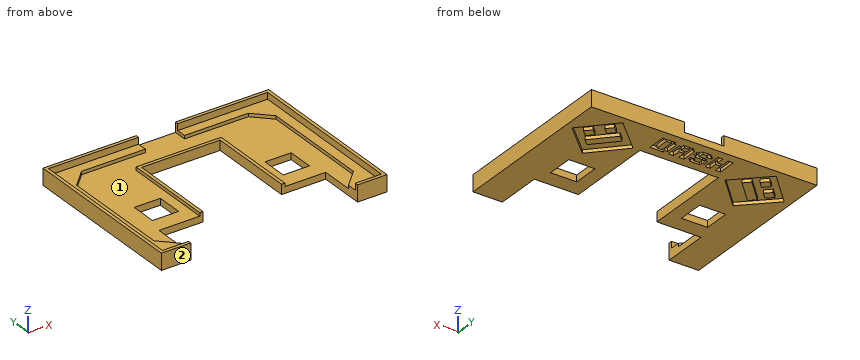
from build123d import *

# Parameters (mm, degrees)
SKICA1_W                    = 67
SKICA1_H                    = 50
P_IDAT_VYSUNUT_M1_DEPTH     = 3
ODEBRAT_VYSUNUT_M1_DEPTH    = 1
SKICA3_W                    = 8
SKICA3_H                    = 8
ODEBRAT_VYSUNUT_M2_DEPTH    = 4
VYSUNOUT_TENKOST_NN_1_DEPTH = 1
VYSUNOUT_TENKOST_NN_2_DEPTH = 5
SKICA6_W                    = 12
SKICA6_H                    = 4
ODEBRAT_VYSUNUT_M3_DEPTH    = 4
ODEBRAT_VYSUNUT_M5_DEPTH    = 1
P_IDAT_START                = -1
P_IDAT_VYSUNUT_M3_DEPTH     = 1
ODEBRAT_VYSUNUT_M7_DEPTH    = 1
SKICA10_W                   = 1.6
SKICA10_H                   = 4
SKICA10_H_2                 = 1.6
P_IDAT_VYSUNUT_M4_DEPTH     = 1


with BuildPart() as part:
    # Skica1 → Přidat vysunutím1 (new body)
    with BuildSketch(Plane.XY):
        Rectangle(SKICA1_W, SKICA1_H)
    extrude(amount=P_IDAT_VYSUNUT_M1_DEPTH)

    # Skica2 → Odebrat vysunutím1 (cut)
    with BuildSketch(Plane.XY.offset(3)):
        Polygon((-25.5, -22), (-30.5, -17), (-30.5, 17), (-25.5, 22), (25.5, 22), (30.5, 17), (30.5, -17), (25.5, -22), align=None)
    extrude(amount=-ODEBRAT_VYSUNUT_M1_DEPTH, mode=Mode.SUBTRACT)

    # Skica3 → Odebrat vysunutím2 (cut, through all)
    with BuildSketch(Plane(origin=(0, 0, 0), x_dir=(-1, 0, 0), z_dir=(0, 0, -1))):
        with Locations((20, -3)):
            Rectangle(SKICA3_W, SKICA3_H)
        with Locations((-20, -3)):
            Rectangle(SKICA3_W, SKICA3_H)
        Polygon((25.5, -25), (-25.5, -25), (-25.5, -12), (-12, -12), (-12, 15), (12, 15), (12, -12), (25.5, -12), align=None)
    extrude(amount=-ODEBRAT_VYSUNUT_M2_DEPTH, mode=Mode.SUBTRACT)

    # Skica4 → Vysunout tenkostěnný1 (add)
    with BuildSketch(Plane.XY.offset(2)):
        Polygon((-12, -12), (-12, 15), (12, 15), (12, -12), (13, -12), (13, 16), (-13, 16), (-13, -12), align=None)
    extrude(amount=VYSUNOUT_TENKOST_NN_1_DEPTH)

    # Skica5 → Vysunout tenkostěnný2 (add)
    with BuildSketch(Plane(origin=(0, 0, 0), x_dir=(-1, 0, 0), z_dir=(0, 0, -1))):
        Polygon((-25.5, -25), (-33.5, -25), (-33.5, 25), (33.5, 25), (33.5, -25), (25.5, -25), (25.5, -26), (34.5, -26), (34.5, 26), (-34.5, 26), (-34.5, -26), (-25.5, -26), align=None)
    extrude(amount=-VYSUNOUT_TENKOST_NN_2_DEPTH)

    # Skica6 → Odebrat vysunutím3 (cut, through all)
    with BuildSketch(Plane.XY.offset(2)):
        with Locations((0, 24)):
            Rectangle(SKICA6_W, SKICA6_H)
    extrude(amount=ODEBRAT_VYSUNUT_M3_DEPTH, mode=Mode.SUBTRACT)

    # Skica7 → Odebrat vysunutím5 (cut)
    with BuildSketch(Plane(origin=(0, 0, 0), x_dir=(-1, 0, 0), z_dir=(0, 0, -1))):
        Polygon((-32.44, 14.540476732), (-23.459523268, 23.94), (-14.06, 14.959523268), (-23.040476732, 5.56), align=None)
        Polygon((14.06, 14.959523268), (23.040476732, 5.56), (32.44, 14.540476732), (23.459523268, 23.94), align=None)
    extrude(amount=-ODEBRAT_VYSUNUT_M5_DEPTH, mode=Mode.SUBTRACT)

    # Skica8 → Přidat vysunutím3 (add)
    with BuildSketch(Plane(origin=(0, 0, 0), x_dir=(-1, 0, 0), z_dir=(0, 0, -1)).offset(P_IDAT_START)):
        Polygon((-29.266904741, 14.966465555), (-27.459304113, 13.239450799), (-25.732289356, 15.047051428), (-27.539889985, 16.774066184), align=None)
        Polygon((-25.467472278, 18.943186938), (-23.659871649, 17.216172182), (-21.932856893, 19.023772811), (-23.740457522, 20.750787567), align=None)
        Polygon((-18.333772811, 16.276666375), (-24.551025932, 9.769304113), (-26.358626561, 11.496318869), (-20.141373439, 18.003681131), align=None)
        Polygon((21.932856893, 19.023772811), (23.740457522, 20.750787567), (25.467472278, 18.943186938), (23.659871649, 17.216172182), align=None)
        Polygon((25.732289356, 15.047051428), (27.539889985, 16.774066184), (29.266904741, 14.966465555), (27.459304113, 13.239450799), align=None)
        Polygon((18.333772811, 16.276666375), (24.551025932, 9.769304113), (26.358626561, 11.496318869), (20.141373439, 18.003681131), align=None)
    extrude(amount=P_IDAT_VYSUNUT_M3_DEPTH)

    # Skica9 → Odebrat vysunutím7 (cut)
    with BuildSketch(Plane(origin=(0, 0, 0), x_dir=(-1, 0, 0), z_dir=(0, 0, -1))):
        Polygon((-10.8, 23.3), (-6.8, 23.3), (-6.8, 22.5), (-6, 22.5), (-6, 18.5), (-6.8, 18.5), (-6.8, 17.7), (-10.8, 17.7), align=None)
        Polygon((-4.4, 23.3), (-1.2, 23.3), (-1.2, 22.5), (-0.4, 22.5), (-0.4, 17.7), (-2, 17.7), (-2, 20.1), (-3.6, 20.1), (-3.6, 17.7), (-5.2, 17.7), (-5.2, 22.5), (-4.4, 22.5), align=None)
        Polygon((1.2, 23.3), (4.4, 23.3), (4.4, 22.5), (5.2, 22.5), (5.2, 21.7), (3.6, 21.7), (3.6, 22.49542164), (2, 22.49542164), (2, 20.89542164), (4.4, 20.89542164), (4.4, 20.09542164), (5.2, 20.09542164), (5.2, 18.5), (4.4, 18.5), (4.4, 17.7), (1.2, 17.7), (1.2, 18.5), (0.4, 18.5), (0.4, 19.3), (2, 19.3), (2, 18.5), (3.6, 18.5), (3.6, 20.09542164), (1.2, 20.09542164), (1.2, 20.9), (0.4, 20.9), (0.4, 22.5), (1.2, 22.5), align=None)
        Polygon((6, 23.3), (7.6, 23.3), (7.6, 20.9), (9.2, 20.9), (9.2, 23.3), (10.8, 23.3), (10.8, 17.7), (9.2, 17.7), (9.2, 20.1), (7.6, 20.1), (7.6, 17.7), (6, 17.7), align=None)
    extrude(amount=-ODEBRAT_VYSUNUT_M7_DEPTH, mode=Mode.SUBTRACT)

    # Skica10 → Přidat vysunutím4 (add)
    with BuildSketch(Plane(origin=(0, 0, 0), x_dir=(-1, 0, 0), z_dir=(0, 0, -1)).offset(P_IDAT_START)):
        with Locations((-8.4, 20.5)):
            Rectangle(SKICA10_W, SKICA10_H)
        with Locations((-2.8, 21.7)):
            Rectangle(SKICA10_W, SKICA10_H_2)
    extrude(amount=P_IDAT_VYSUNUT_M4_DEPTH)


solid = part.part
Source: CAD feature listing. Evaluate the final solid. Frame: model axes, mm. Face numbers are marked on the shaded views. Give positions to 0.01 mm unless a question says otherwise; leave off trailing zeros. Write each loop counter-clockwise with the first axis right and the second up, starting at its lowest first coordinate (ties: lowest second). Pieces come first, ordered by that corner, then holes. Notation, with made-up numbers: M -38,15 L -17,15 A11 cw -17,23 Z; hole C 26.5,66.25 d2. An arc over 180 degrees is marked long. Return JSON: item names as keys, results as strings. Group by question number.
1) Cut plane B-B, the plane z = 3.8. Output: boundary loops of the cut face in (x, y).
2) Material intervals for line 1 along X through (y, z) = (-1, 0.3); line 2 along X through (y, z) = (13, 2.9); line 3 along X through (y, z) = (-11.5, 1.1), sorted ascending. Write a range as [from, to].
3) Cut plane A-A, the plane y = -20. Output: boundary loops of the cut face in (x, z).
4) Pull-direction query (X, two-part tool) for the marked faces 1 and 2; classes: pulls with the +X half, pulls with the -X half, needs draft (parallel to the pull), parting line crosses it, or undercut.
5) Pin query (flat end, axial travel): P1, Ø0.9, axis at x = 6.5, z = 0.5, coming from the -Y side; P2, Ø2, axis at x = 21.5, z = 1.5, coming from the -Y side; P3, Ø8, axis at x = 24.5, y = -19, coming from the +Z side. Return the tip coordinate at first contact, or that it passes through.
6) Cut plane C-C, the plane y = -9. Output: boundary loops of the cut face in (x, z).
Recorded:
{
 "1": {"outline": "M -34.5,-26 L -25.5,-26 L -25.5,-25 L -33.5,-25 L -33.5,25 L -6,25 L -6,26 L -34.5,26 Z; M 6,25 L 33.5,25 L 33.5,-25 L 25.5,-25 L 25.5,-26 L 34.5,-26 L 34.5,26 L 6,26 Z"},
 "2": {"line 1": "x = [-34.5, -24], [-16, -12], [12, 16], [24, 34.5]", "line 2": "x = [-34.5, -30.5], [-13, -12], [12, 13], [30.5, 34.5]", "line 3": "x = [-34.5, -12], [12, 34.5]"},
 "3": {"outline": "M -34.5,0 L -25.5,0 L -25.5,2 L -27.5,2 L -27.5,3 L -33.5,3 L -33.5,5 L -34.5,5 Z; M 25.5,0 L 34.5,0 L 34.5,5 L 33.5,5 L 33.5,3 L 27.5,3 L 27.5,2 L 25.5,2 Z"},
 "4": {"face 1": "undercut", "face 2": "needs draft"},
 "5": {"P1": "stops at y = 15", "P2": "stops at y = -12", "P3": "stops at z = 3"},
 "6": {"outline": "M -34.5,0 L -12,0 L -12,3 L -13,3 L -13,2 L -30.5,2 L -30.5,3 L -33.5,3 L -33.5,5 L -34.5,5 Z; M 12,0 L 34.5,0 L 34.5,5 L 33.5,5 L 33.5,3 L 30.5,3 L 30.5,2 L 13,2 L 13,3 L 12,3 Z"}
}
